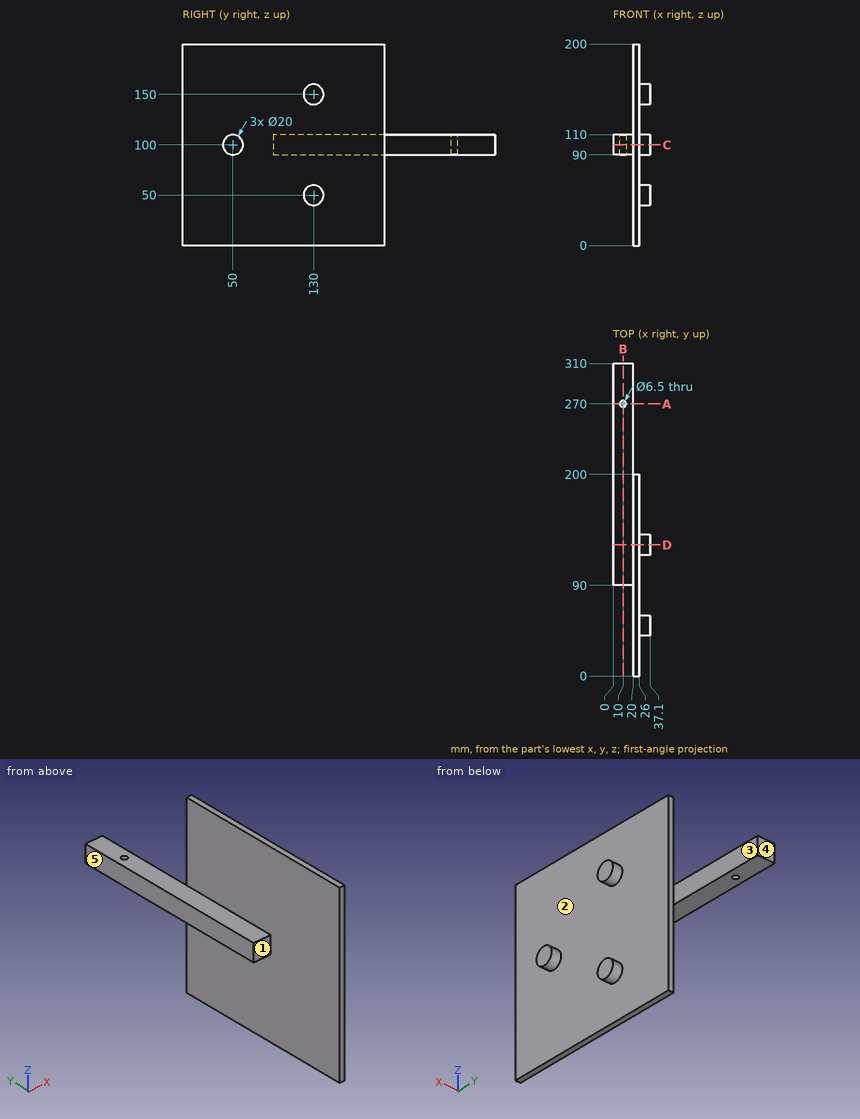
Study the drawing (mm; zero at the part's minimum x, y, z) and answer. A direction names the side the tool comes from. Coordinates: 2 decimals unless noted, no trailing zeros. Write each loop counter-clockwise with the first axis right and the second up, starting at its lowest first coordinate (ties: lowest second). Pieces come first, ordered by that corner, then holes. Notation, with made-up numbers: (-5.75, 59.25) - (29.25, 59.25) arc R17 ccw to (29.25, 68.25) - close; hole circle Ø4 at (41, -2). An arc over 180 degrees is marked (long way). One line per item, written item: value.
1) Find section D-D (y = 130). Give the vertices of the cut face in (x, z).
Geometry check:
outline: (0, 90) - (20, 90) - (20, 0) - (26, 0) - (26, 40) - (37.1, 40) - (37.1, 60) - (26, 60) - (26, 140) - (37.1, 140) - (37.1, 160) - (26, 160) - (26, 200) - (20, 200) - (20, 110) - (0, 110) - close
2) Find section C-C (z = 100). Give the vertices of the cut face in (x, y), and give its area (3 significant figures).
Geometry check:
outline: (0, 90) - (20, 90) - (20, 0) - (26, 0) - (26, 40) - (37.1, 40) - (37.1, 60) - (26, 60) - (26, 200) - (20, 200) - (20, 310) - (0, 310) - close; hole circle Ø6.5 at (10, 270)
area: 5,790 mm2
3) Consider line 1 along X through (y, z) = (270, 96); line 2 along Y through (x, z) = (10, 104.5); line 3 along Z through (x, y) = (8, 106.5). Determine where each line is inside the solid, lowest interval first. Write a range as from..to.
Geometry check:
line 1: x = 0..6.75, 13.25..20
line 2: y = 90..266.75, 273.25..310
line 3: z = 90..110
4) A tool of negligible diameter and unlimited length cuts with its end or side. For the marked faces 1, 2, 3, 4 and 5, from which of +Z, -Z, +X, -X, +Y, -Y can it reach the whole face along a straight path? Write none if from no direction.
Geometry check:
face 1: +Z, -Z, -X, -Y
face 2: +X
face 3: +Z, -Z, +X, +Y
face 4: +Z, -Z, +X, -X, +Y
face 5: +Z, -Z, -X, +Y, -Y
5) Find section A-A (y = 270). Give the vertices of the cut face in (x, z), and give its area (3 significant figures).
Geometry check:
outline: (0, 90) - (6.75, 90) - (6.75, 110) - (0, 110) - close; (13.25, 90) - (20, 90) - (20, 110) - (13.25, 110) - close
area: 270 mm2
6) Each of these flat-tipped pins is pushed along its axis until it touches: pin 1 Ø6 at (x, y) = (19.5, 250) entering from -Z; pin 2 Ø6 at (x, y) = (17.5, 213) entering from +Z; pin 3 Ø10 at (x, z) = (30.5, 125.5) entering from -Y; pin 4 Ø22 at (x, z) = (7.5, 96) entering from -Y. Where does it stop, or does it pass through?
Geometry check:
pin 1: stops at z = 90
pin 2: stops at z = 110
pin 3: stops at y = 0
pin 4: stops at y = 90
7) Find section B-B (x = 10). Give the vertices of the cut face in (y, z), and give its area (3 significant figures).
Geometry check:
outline: (90, 90) - (266.75, 90) - (266.75, 110) - (90, 110) - close; (273.25, 90) - (310, 90) - (310, 110) - (273.25, 110) - close
area: 4,270 mm2
